The listing builds one solid part. Answer for the finished solid, in the listing's coordinates (mm). Face numbers are marked on the shaded views. Round coordinates to 2 decimals unless told otherwise and drop trailing zeros. Loops run counter-clockwise (first coordinate to the right, second up) from the corner with the lowest first, then second, coordinate; pieces in that order, holes last. Notation, with made-up numbers: (-20, 78) - (32, 78) arc R12 ccw to (32, 91) - close; hole circle Ø4 at (64, 88.25). An arc over 180 degrees is marked (long way). One line per question, with ' | ' between items. Start each with the question number.
from build123d import *

# Parameters (mm, degrees)
PAD_DEPTH       = 10
SKETCH001_W     = 3.935465
SKETCH001_H     = 80.004486
POCKET_DEPTH    = 10.001
POCKET001_DEPTH = 10.001


with BuildPart() as part:
    # Sketch → Pad (new body)
    with BuildSketch(Plane.XY):
        with BuildLine():
            ThreePointArc((30, -40), (0, 50), (-30, -40))
            Line((-30, -133.787827), (-30, -40))
            Line((30, -133.787827), (-30, -133.787827))
            Line((30, -40), (30, -133.787827))
        make_face()
        with BuildLine():
            Line((5.320689, -2.850805), (5.546297, 10))
            Line((5.546297, 10), (27.430071, 20))
            ThreePointArc((5.320689, -2.850805), (22.53342, 2.616363), (27.430071, 20))
        make_face(mode=Mode.SUBTRACT)
        with BuildLine():
            Line((-5.320689, -2.850805), (-5.546297, 10))
            Line((-5.546297, 10), (-27.430071, 20))
            ThreePointArc((-27.430071, 20), (-22.53342, 2.616363), (-5.320689, -2.850805))
        make_face(mode=Mode.SUBTRACT)
    extrude(amount=PAD_DEPTH)

    # Sketch001 → Pocket (cut, through all)
    with BuildSketch(Plane.XY.offset(10)):
        with Locations((-21.967733, -90.002243)):
            Rectangle(SKETCH001_W, SKETCH001_H)
        with Locations((-8.032267, -90.002243)):
            Rectangle(SKETCH001_W, SKETCH001_H)
        with Locations((5.903197, -90.002243)):
            Rectangle(SKETCH001_W, SKETCH001_H)
        with Locations((19.838662, -90.002243)):
            Rectangle(SKETCH001_W, SKETCH001_H)
    extrude(amount=-POCKET_DEPTH, mode=Mode.SUBTRACT)

    # Sketch002 → Pocket001 (cut, through all)
    with BuildSketch(Plane.XY.offset(10)):
        Polygon((-10, -16.418013), (-2.0219, -20), (-5.526516, -30), align=None)
        Polygon((10, -16.418013), (2.0219, -20), (5.526516, -30), align=None)
    extrude(amount=-POCKET001_DEPTH, mode=Mode.SUBTRACT)


solid = part.part
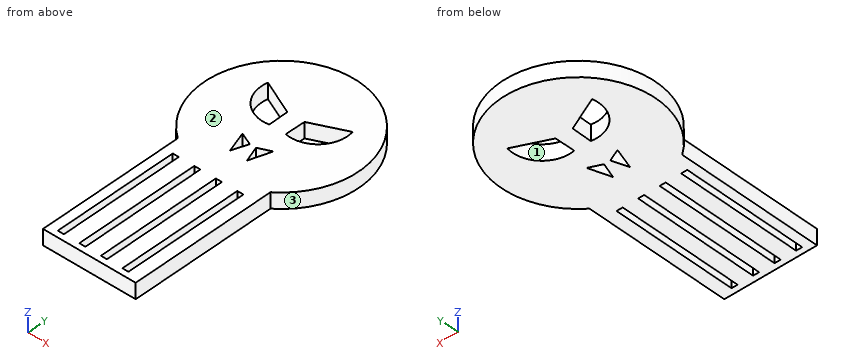
(1) Determine the mould class of the marked faces 1, 2 and 3 for opening direction Y: pulls with the +Y half, pulls with the -Y half, needs draft (parallel to the pull), parting line crosses it, or undercut.
(2) Find section A-A on y = -60. Write down the section's boundary in (x, z), plus the area to 3 significant figures.
(3) Each of these flat-tipped pins is pushed along its axis until it touches: P1, Ø5, axis at y = -74, z = 4, coming from the +X side; P2, Ø1.2, axis at x = -21.5, z = 6, coming from the +Y side; P3, Ø4.5, axis at x = 6, z = 5.5, coming from the +Y side. Where does it stop, or does it pass through?
(4) Find section B-B on y = 0. Write down the section's boundary in (x, z), plus the area to 3 significant figures.
(5) Find section C-C on x = 37. Write down the section's boundary in (y, z), plus the area to 3 significant figures.
(6) Consider L1, parallel to X at y = -110.5, z = 6; L2, parallel to X at y = 11, z = 8.5 (3 decimals); L3, parallel to X at y = 13.5, z = 1.5. Determine where each line is inside the solid, lowest interval first.
Answer below:
1) face 1: undercut | face 2: needs draft | face 3: parting line crosses it
2) outline: (-30, 0) - (-23.94, 0) - (-23.94, 10) - (-30, 10) - close; (-20, 0) - (-10, 0) - (-10, 10) - (-20, 10) - close; (-6.06, 0) - (3.94, 0) - (3.94, 10) - (-6.06, 10) - close; (7.87, 0) - (17.87, 0) - (17.87, 10) - (7.87, 10) - close; (21.81, 0) - (30, 0) - (30, 10) - (21.81, 10) - close | area: 443 mm2
3) P1: x = 30 | P2: y = 45.42 | P3: y = 49.86
4) outline: (-50, 0) - (-19.39, 0) - (-19.39, 10) - (-50, 10) - close; (-5.37, 0) - (5.37, 0) - (5.37, 10) - (-5.37, 10) - close; (19.39, 0) - (50, 0) - (50, 10) - (19.39, 10) - close | area: 720 mm2
5) outline: (-33.63, 0) - (33.63, 0) - (33.63, 10) - (-33.63, 10) - close | area: 673 mm2
6) L1: -30 to -23.94, -20 to -10, -6.06 to 3.94, 7.87 to 17.87, 21.81 to 30 | L2: -48.775 to -27.259, -7.735 to 7.735, 27.259 to 48.775 | L3: -48.14 to -27.74, -13.21 to 13.21, 27.74 to 48.14
